The drawing under review shows one solid part. Ordinate dimensions are in mm from its lowest x, y, z. A direction names the side the tool comes from. Round coordinates to 2 decimals unless told otherwise and drop trailing zeros. Write each loop counter-clockwise with the first axis right and the second up, starting at its lowest first coordinate (ties: lowest second). Pieces come first, ordered by that corner, then holes.
Item 1: Add section D-D (x = 9.5). Give the boundary of the cut face in (y, z).
Item 2: To check wall thickness, follow L1, parallel to Y at x = 10, z = 1.1; L2, parallel to Y at x = 20, z = 1; L3, parallel to Z at x = 28.5, y = 27. State the ranges of each line that lie inside material, in increasing order.
Item 3: Add section B-B (x = 20). Give the boundary of the cut face in (y, z).
Item 4: Add section A-A (y = 37.5). Give the boundary of the cut face in (x, z) (1 decimal).
Item 5: Machinability: for the marked faces 1 and 2, which of the approach directions +Z, -Z, +X, -X, +Y, -Y give a long, thin tool a straight path to every point of the face, cutting with its end or side? Answer none if there is none.
Item 6: Add section C-C (z = 1.15). Give the boundary of the cut face in (x, y), plus the area to 3 significant figures.
Item 7: Clearance check with flat-ended pins moving along their axes: pin 1 Ø1 at (y, z) = (35, 3) entering from +X; pin 2 Ø3.5 at (x, y) = (20, 30) entering from +Z; pin 3 Ø3 at (y, z) = (16, 3.5) entering from +X; pin 4 Ø2.5 at (x, y) = (10, 22.5) entering from +Z. State where each tip first meets the part, or that it passes through.
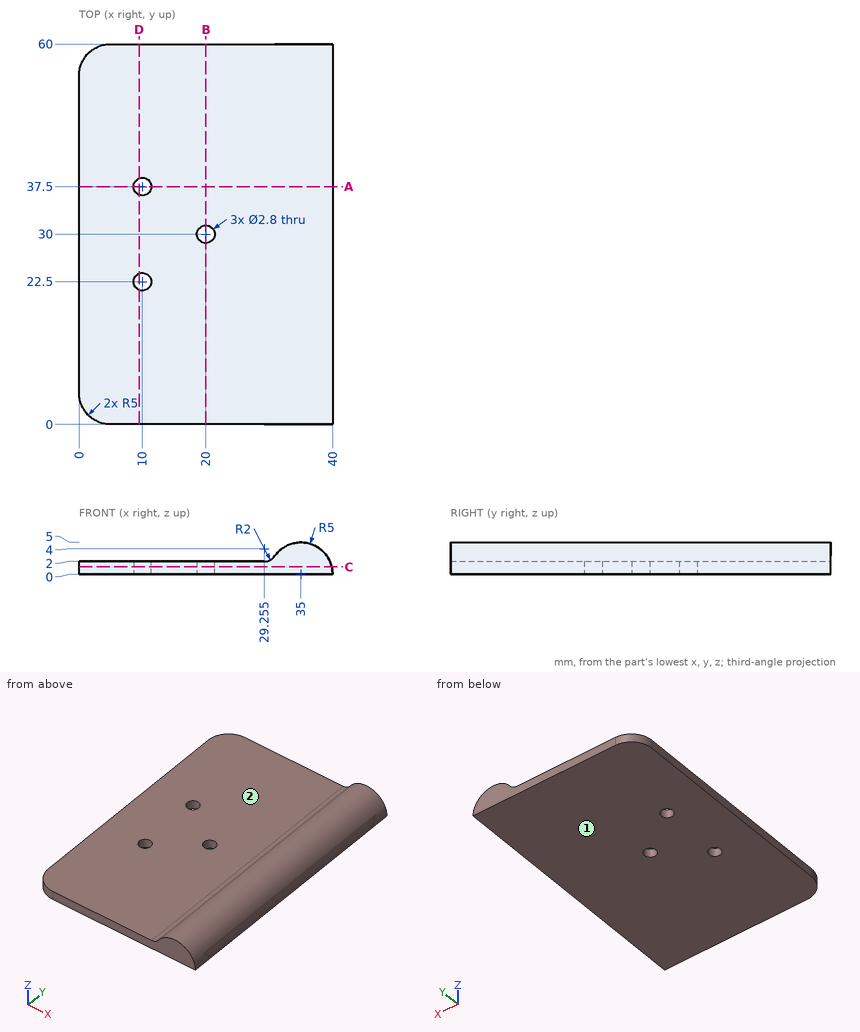
Numbers:
1. outline: (0, 0) - (21.19, 0) - (21.19, 2) - (0, 2) - close; (23.81, 0) - (36.19, 0) - (36.19, 2) - (23.81, 2) - close; (38.81, 0) - (60, 0) - (60, 2) - (38.81, 2) - close
2. L1: y = 0 to 21.1, 23.9 to 36.1, 38.9 to 60
2. L2: y = 0 to 28.6, 31.4 to 60
2. L3: z = 0 to 2
3. outline: (0, 0) - (28.6, 0) - (28.6, 2) - (0, 2) - close; (31.4, 0) - (60, 0) - (60, 2) - (31.4, 2) - close
4. outline: (0, 0) - (8.6, 0) - (8.6, 2) - (0, 2) - close; (11.4, 0) - (40, 0) arc R5 ccw to (30.9, 2.9) arc R2 cw to (29.3, 2) - (11.4, 2) - close
5. face 1: -Z, +X, -X, +Y, -Y
5. face 2: +Z, -X, +Y, -Y
6. outline: (0, 5) arc R5 ccw to (5, 0) - (39.87, 0) - (39.87, 60) - (5, 60) arc R5 ccw to (0, 55) - close; hole circle Ø2.8 at (10, 22.5); hole circle Ø2.8 at (10, 37.5); hole circle Ø2.8 at (20, 30)
6. area: 2,360 mm2
7. pin 1: stops at x = 39.33
7. pin 2: stops at z = 2
7. pin 3: stops at x = 39.58
7. pin 4: passes through
